Input: part model. Units: mm. Frame: model coordinates. Face numbers are marked on the shaded views. A direction names the side the tool comes from. Coordinates: 2 decimals unless noted, no trailing zeros. Order: outer loops, then holes, each group sorted by start corner. A loop starts at its lowest first (then second) coordinate and runs counter-clockwise, first axis right, second up. Notation, with made-up numbers: (31.25, -2.75) - (57.25, -2.75) arc R22 cw to (57.25, 6.25) - close; hole circle Ø4 at (-22, 58). An arc over 180 degrees is marked (long way). One line per question, with ' | ' between items.
from build123d import *

# Parameters (mm, degrees)
SKETCH_1_W          = 16.31456143534598
SKETCH_1_H          = 26.000000000000004
SKETCH_1_R          = 0.7500000000000021
EXTRUDE_1_DEPTH     = 14.5
SKETCH_2_R          = 33
CUT_EXTRUDE_1_DEPTH = 11.75
CUT_EXTRUDE_2_DEPTH = 2
CUT_EXTRUDE_7_REACH = 50.021
SKETCH_8_R          = 22
FILLET_1_R          = 1
CHAMFER_1_SIZE      = 1
SKETCH_4_R          = 1.2500000000000002
SKETCH_4_R_2        = 1.2499999999999991
CUT_EXTRUDE_3_DEPTH = 1.5
SKETCH_5_R          = 0.7500000000000004
CUT_EXTRUDE_4_DEPTH = 25.169333290066117
CUT_EXTRUDE_5_REACH = 50.021
FILLET_2_R          = 3
CHAMFER_3_SIZE      = 1
SKETCH_7_R          = 1.949999999999999
CUT_EXTRUDE_6_DEPTH = 1
CHAMFER_4_SIZE      = 1


with BuildPart() as part:
    # Эскиз1 → Бобышка-Вытянуть1 (new, symmetric)
    with BuildSketch(Plane(origin=(0, 0, 0), x_dir=(1, 0, 0), z_dir=(0, 1, 0))):
        with Locations((27.84271928232701, 0)):
            Rectangle(SKETCH_1_W, SKETCH_1_H)
        with Locations(Location((23.68543856465402, -8, 0), (0, 0, 90))):
            Circle(SKETCH_1_R, mode=Mode.SUBTRACT)
        with Locations(Location((23.68543856465402, 8, 0), (0, 0, 90))):
            Circle(SKETCH_1_R, mode=Mode.SUBTRACT)
    extrude(amount=EXTRUDE_1_DEPTH, both=True)

    # Эскиз2 → Вырез-Вытянуть1 (cut, symmetric)
    with BuildSketch(Plane(origin=(0, 0, 0), x_dir=(1, 0, 0), z_dir=(0, 1, 0))):
        Circle(SKETCH_2_R)
    extrude(amount=CUT_EXTRUDE_1_DEPTH, both=True, mode=Mode.SUBTRACT)

    # Эскиз3 → Вырез-Вытянуть2 (cut)
    with BuildSketch(Plane(origin=(36, 0, 0), x_dir=(0, 0, -1), z_dir=(1, 0, 0))):
        Polygon((-13.000000000000004, 10.999999999999998), (-5.000000000000003, 10.999999999999996), (-5.000000000000002, 4.699999999999998), (0.5999999999999969, 4.699999999999999), (0.5999999999999981, -4.699999999999999), (-5.000000000000001, -4.7), (-5, -10.999999999999996), (-13, -11.000000000000002), align=None)
    extrude(amount=-CUT_EXTRUDE_2_DEPTH, mode=Mode.SUBTRACT)

    # Эскиз8 → Вырез-Вытянуть7 (cut, up to next)
    with BuildSketch(Plane(origin=(0, 14.5, 0), x_dir=(1, 0, 0), z_dir=(0, 1, 0)), mode=Mode.PRIVATE) as cut_extrude_7_sk1:
        Circle(SKETCH_8_R)
    cut_extrude_7_tool1 = extrude(cut_extrude_7_sk1.sketch, amount=-CUT_EXTRUDE_7_REACH, mode=Mode.PRIVATE) & part.part
    add(cut_extrude_7_tool1.solids().sort_by_distance((0, 14.5, 0))[0], mode=Mode.SUBTRACT)

    # Скругление1
    fillet_1_edges = [part.edges().sort_by_distance(p)[0] for p in [
        (35, 10.999999999999996, 5.000000000000003),
        (35, -10.999999999999996, 5),
    ]]
    fillet(fillet_1_edges, radius=FILLET_1_R)

    # Фаска1
    chamfer_1_edges = [part.edges().sort_by_distance(p)[0] for p in [
        (35, 4.699999999999999, -0.5999999999999969),
        (35, -4.699999999999999, -0.5999999999999981),
    ]]
    chamfer(chamfer_1_edges, length=CHAMFER_1_SIZE)

    # Эскиз4 → Вырез-Вытянуть3 (cut)
    with BuildSketch(Plane(origin=(33.99999999999999, 0, 0), x_dir=(0, 0, -1), z_dir=(1, 0, 0))):
        with Locations((-4.300000000000002, 0)):
            Circle(SKETCH_4_R)
        with Locations((-10.700000000000001, 0)):
            Circle(SKETCH_4_R_2)
    extrude(amount=-CUT_EXTRUDE_3_DEPTH, mode=Mode.SUBTRACT)

    # Эскиз5 → Вырез-Вытянуть4 (cut, through all)
    with BuildSketch(Plane(origin=(33.99999999999999, 0, 0), x_dir=(0, 0, -1), z_dir=(1, 0, 0))):
        with Locations((-9.500000000000002, 7.5)):
            Circle(SKETCH_5_R)
        with Locations((-9.500000000000002, -7.5)):
            Circle(SKETCH_5_R)
    extrude(amount=-CUT_EXTRUDE_4_DEPTH, mode=Mode.SUBTRACT)

    # Эскиз6 → Вырез-Вытянуть5 (cut, up to next)
    with BuildSketch(Plane.XZ.offset(14.5), mode=Mode.PRIVATE) as cut_extrude_5_sk1:
        with BuildLine():
            ThreePointArc((25, -3.5), (21.5, 4.3e-16), (25, 3.5))
            Line((25, 3.5), (19.68543856465402, 3.499999999999999))
            Line((19.68543856465402, 3.499999999999999), (19.68543856465402, -3.500000000000001))
            Line((19.68543856465402, -3.500000000000001), (25, -3.5))
        make_face()
    cut_extrude_5_tool1 = extrude(cut_extrude_5_sk1.sketch, amount=-CUT_EXTRUDE_5_REACH, mode=Mode.PRIVATE) & part.part
    # Эскиз6 → Вырез-Вытянуть5 (cut, up to next)
    with BuildSketch(Plane.XZ.offset(14.5), mode=Mode.PRIVATE) as cut_extrude_5_sk2:
        with BuildLine():
            ThreePointArc((28.5, 0), (27.474873734152915, 2.474873734152916), (25, 3.5))
            Line((25, 3.5), (25, -3.5))
            ThreePointArc((25, -3.5), (27.474873734152915, -2.474873734152917), (28.5, -8.6e-16))
        make_face()
    cut_extrude_5_tool2 = extrude(cut_extrude_5_sk2.sketch, amount=-CUT_EXTRUDE_5_REACH, mode=Mode.PRIVATE) & part.part
    # Эскиз6 → Вырез-Вытянуть5 (cut, up to next)
    with BuildSketch(Plane.XZ.offset(14.5), mode=Mode.PRIVATE) as cut_extrude_5_sk3:
        with BuildLine():
            Line((25, -3.5), (25, 3.5))
            ThreePointArc((25, 3.5), (21.5, 4.3e-16), (25, -3.5))
        make_face()
    cut_extrude_5_tool3 = extrude(cut_extrude_5_sk3.sketch, amount=-CUT_EXTRUDE_5_REACH, mode=Mode.PRIVATE) & part.part
    # Эскиз6 → Вырез-Вытянуть5 (cut, up to next)
    with BuildSketch(Plane.XZ.offset(14.5), mode=Mode.PRIVATE) as cut_extrude_5_sk4:
        with BuildLine():
            ThreePointArc((28.5, 0), (27.474873734152915, 2.474873734152916), (25, 3.5))
            Line((25, 3.5), (25, -3.5))
            ThreePointArc((25, -3.5), (27.474873734152915, -2.474873734152917), (28.5, -8.6e-16))
        make_face()
    cut_extrude_5_tool4 = extrude(cut_extrude_5_sk4.sketch, amount=-CUT_EXTRUDE_5_REACH, mode=Mode.PRIVATE) & part.part
    # Эскиз6 → Вырез-Вытянуть5 (cut, up to next)
    with BuildSketch(Plane.XZ.offset(14.5), mode=Mode.PRIVATE) as cut_extrude_5_sk5:
        with BuildLine():
            Line((25, -3.5), (25, 3.5))
            ThreePointArc((25, 3.5), (21.5, 4.3e-16), (25, -3.5))
        make_face()
    cut_extrude_5_tool5 = extrude(cut_extrude_5_sk5.sketch, amount=-CUT_EXTRUDE_5_REACH, mode=Mode.PRIVATE) & part.part
    add(cut_extrude_5_tool1.solids().sort_by_distance((21.087199, -14.5, 0))[0], mode=Mode.SUBTRACT)
    add(cut_extrude_5_tool2.solids().sort_by_distance((26.485446, -14.5, 0))[0], mode=Mode.SUBTRACT)
    add(cut_extrude_5_tool3.solids().sort_by_distance((23.514554, -14.5, 0))[0], mode=Mode.SUBTRACT)
    add(cut_extrude_5_tool4.solids().sort_by_distance((26.485446, -14.5, 0))[0], mode=Mode.SUBTRACT)
    add(cut_extrude_5_tool5.solids().sort_by_distance((23.514554, -14.5, 0))[0], mode=Mode.SUBTRACT)

    # Скругление2
    fillet_2_edges = [part.edges().sort_by_distance(p)[0] for p in [
        (19.68543856465402, 13.125, -13),
        (19.68543856465402, 13.125, 13),
        (19.68543856465402, -13.125, -13),
        (19.68543856465402, -13.125, 13),
        (36, 0, -13),
        (36, 12.75, 13),
        (19.68543856465402, -13.125, 3.499999999999999),
        (19.68543856465402, -13.125, -3.500000000000001),
    ]]
    fillet(fillet_2_edges, radius=FILLET_2_R)

    # Фаска3
    chamfer_3_edges = [part.edges().sort_by_distance(p)[0] for p in [
        (23.84271928232701, -14.5, -3.5),
        (28.5, -14.5, -2.56e-15),
        (23.84271928232701, -14.5, 3.5),
        (19.68543856465402, -14.5, 8.25),
        (19.68543856465402, -14.5, -8.25),
        (27.84271928232701, -14.5, -13),
        (36, -14.5, 0),
        (27.84271928232701, -14.5, 13),
        (35.121320343559645, -14.5, 12.121320343559642),
        (35.121320343559645, -14.5, -12.121320343559642),
        (20.56411822109438, -14.5, 12.121320343559642),
        (20.56411822109438, -14.5, -12.121320343559642),
        (20.56411822109438, -14.5, -4.378679656440358),
        (20.56411822109438, -14.5, 4.378679656440358),
        (19.68543856465402, 14.5, -9.911300960978625),
        (27.84271928232701, 14.5, -13),
        (27.84271928232701, 14.5, 13),
        (36, 14.5, 0),
        (35.121320343559645, 14.5, 12.121320343559642),
        (35.121320343559645, 14.5, -12.121320343559642),
        (20.56411822109438, 14.5, 12.121320343559642),
        (20.56411822109438, 14.5, -12.121320343559642),
        (19.68543856465402, 14.5, 9.911300960978625),
    ]]
    chamfer(chamfer_3_edges, length=CHAMFER_3_SIZE)

    # Эскиз7 → Вырез-Вытянуть6 (cut)
    with BuildSketch(Plane(origin=(0, 14.5, 0), x_dir=(1, 0, 0), z_dir=(0, 1, 0))):
        with Locations(Location((23.68543856465402, 8, 0), (0, 0, 270))):
            Circle(SKETCH_7_R)
        with Locations(Location((23.68543856465402, -8, 0), (0, 0, 270))):
            Circle(SKETCH_7_R)
    cut_extrude_6 = extrude(amount=-CUT_EXTRUDE_6_DEPTH, mode=Mode.SUBTRACT)

    # Зеркальное отражение1: Вырез-Вытянуть6 across plane
    add(cut_extrude_6.mirror(Plane.ZX), mode=Mode.SUBTRACT)

    # Фаска4
    # the kernel refuses this chamfer: 1 mm, written as the material it takes off along each edge
    with BuildSketch(Plane(origin=(0, 14.5, 0), x_dir=(0.8941152756835695, 0, -0.44783688301578556), z_dir=(-0.44783688301578556, 0, -0.8941152756835695))) as chamfer_4_piece_1:
        Polygon((21.999999999999993 + CHAMFER_4_SIZE, 0), (21.999999999999996, CHAMFER_4_SIZE), (21.999999999999993, 0), align=None)
    revolve(axis=Axis((0, 14.5, 0), (0, -1, 0)), revolution_arc=53.209970164509144, mode=Mode.SUBTRACT)


solid = part.part
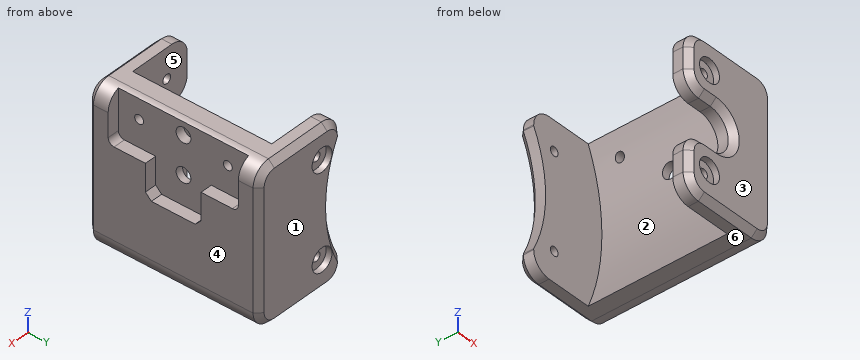
Item 1: Section C-C on y = 6.25. Return the cut outline in (x, z), and give its area (3 significant figures).
Data:
outline: (30.33, -13) - (33, -13) arc R3 ccw to (36, -10) - (36, 5) - (34, 5) - (34, 12.83) arc R3 ccw to (33, 13) - (30.33, 13) arc R33 cw to start | area: 82.8 mm^2
Item 2: Access query for the marked faces 5 and 6. Directions: +Z, -Z, +X, -X, +Y, -Y. A direction counts if a zero-diameter tool reaches every point of the face in a straight line with its end or side. Return the directions, or none.
Data:
face 5: -X | face 6: -Z, +X, -X, +Y, -Y
Item 3: Section D-D on x = 26. Count the separate pieces of the cut face and the enclosed holes in it, and give its area (3 significant figures).
Data:
separate pieces: 3 | enclosed holes: 0 | area: 122 mm^2
Item 4: Section A-A on y = 0. Return the cut outline in (x, z).
Data:
outline: (30.33, -13) - (33, -13) arc R3 ccw to (36, -10) - (36, -0.6) - (34, -0.6) - (34, 3.05) - (32.86, 3.05) arc R33 cw to start; (30.33, 13) arc R33 cw to (32.53, 5.55) - (34, 5.55) - (34, 9.45) - (32.5, 9.45) - (32.5, 11.95) - (34, 11.95) - (34, 12.83) arc R3 ccw to (33, 13) - close
Item 5: Draft query along Y for the marked faces 1, 2, 3 and 4. Return one class per face: released by +Y, released by -Y, zero draft, split by the parting line, or undercut.
Data:
face 1: released by +Y | face 2: undercut | face 3: released by -Y | face 4: zero draft
Item 6: Ray query, line 1 (Y direction, x = 33.15, z = 4.3); line 2 (Y direction, x = 31.75, z = 2.5); line 3 (X direction, y = -12.6, z = 8). Return the intervals inside material, ascending.
Data:
line 1: -14.5 to -1.25, 1.25 to 14.5 | line 2: -14.5 to -11.75, 11.75 to 14.5 | line 3: 19.69 to 22.94, 24.44 to 36
Item 7: Section B-B on z = 0. Return the cut outline in (x, y), and give its area (3 significant figures).
Data:
outline: (22, 11.75) - (33, 11.75) - (33, -11.75) - (28.5, -11.75) - (28.5, -13.5) - (29.5, -14.5) - (35, -14.5) - (36, -13.5) - (36, -4.3) - (34, -4.3) - (34, 4.3) - (36, 4.3) - (36, 13.5) - (35, 14.5) - (23, 14.5) - (22, 13.5) - close | area: 110 mm^2
Item 8: Contact query for flat-ended pins moving along their axis: P1, Ø1.2, axis at x = 23.69, z = 8, coming from the -Y side; P2, Ø2, axis at x = 23.69, z = 8, coming from the +Y side; P3, Ø1.2, axis at y = 0.5, z = 10, coming from the +X side; P4, Ø0.6, axis at x = 35, y = 7, coming from the +Z side. Output: stop coordinate, or through.
Data:
P1: through | P2: y = 13.5 | P3: x = 34 | P4: z = 5
